The model under review builds one solid part; all positions refer to its coordinate system, in mm. A direction names the side the tool comes from. Give positions to 0.01 mm unless a question says otherwise; leave off trailing zeros. Order: outer loops, then holes, each group sorted by start corner. A loop starts at its lowest first (then second) coordinate and runs counter-clockwise, first axis right, second up. Notation, with made-up numbers: (58.5, -7.5) - (83.5, -7.5) arc R23 ccw to (83.5, 18.5) - close; hole circle Ø8 at (14.25, 61). An arc over 180 degrees is marked (long way). Answer as CSV lines item,"result". Start each with the question number.
from build123d import *

# Parameters (mm, degrees)
F0_W     = 152.4
F0_H     = 76.2
F1_DEPTH = 12.7
F2_R     = 6.35
F2_R_2   = 5.9938939969
F2_R_3   = 6.6713502792
F2_R_4   = 7.8689754044
F3_DEPTH = 12.7
F4_W     = 25.4
F4_H     = 50.8
F6_W     = 17.78
F6_H     = 17.78
F8_R     = 5.08
F9_SIZE  = 5.08


with BuildPart() as f1:
    # F0 (on Top) → F1 (new body)
    with BuildSketch(Plane.XY):
        Rectangle(F0_W, F0_H)
    extrude(amount=F1_DEPTH)

    # F2 (on Top) → F3 (cut)
    with BuildSketch(Plane.XY):
        with Locations((-67.2256079361, 27.7522747686)):
            Circle(F2_R)
        with Locations((-68.6647296343, -27.1399345782)):
            Circle(F2_R_2)
        with Locations((60.0338615502, 30.0137525229)):
            Circle(F2_R_3)
        with Locations((64.9679941536, -26.7287574834)):
            Circle(F2_R_4)
    extrude(amount=F3_DEPTH, mode=Mode.SUBTRACT)

    # F4 (on Front) → F5 (revolve)
    with BuildSketch(Plane.XZ):
        with Locations((-12.7, 38.1)):
            Rectangle(F4_W, F4_H)
    revolve(axis=Axis((0, 0, 38.1), (0, 0, -1)))

    # F6 (on Front) → F7 (revolve, cut)
    with BuildSketch(Plane.XZ):
        with Locations((21.59, 41.91)):
            Rectangle(F6_W, F6_H)
    revolve(axis=Axis((0, 0, 63.5), (0, 0, -1)), mode=Mode.SUBTRACT)

    # F8
    f8_edges = [f1.edges().sort_by_distance(p)[0] for p in [
        (25.4, 0, 63.5),
        (25.4, 0, 12.7),
    ]]
    fillet(f8_edges, radius=F8_R)

    # F9
    f9_edges = [f1.edges().sort_by_distance(p)[0] for p in [
        (25.4, 0, 33.02),
        (25.4, 0, 50.8),
    ]]
    chamfer(f9_edges, length=F9_SIZE)


solid = f1.part
Item 1: For line 1 along Z through (x, y) = (45.5, -10); line 2 along X through (y, z) = (26.5, 4); line 3 along Z through (x, y) = (-15.5, 9.5), list the stretches that pass through material, from the lowest coordinate up.
Item 2: Machinability: for faces 5 (the face through (5.506, -24.796, 57.168)), 6 (the face through (-1, -38.1, 6)), 7 (the face through (0, 13, 33.02)), which of the approach directions +Z, -Z, +X, -X, +Y, -Y give a long, thin tool a straight path to every point of the face, cutting with its end or side? Answer none if there is none.
Item 3: Clearance check with flat-ended pins moving along their axes: pin 1 (10 mm diameter, centred on x = -53.5, y = 12, fed in from +Z); pin 2 (20.5 mm diameter, centred on x = -0.5, y = 2, fed in from -Z); pin 3 (10 mm diameter, centred on y = 14.5, z = 49, fed in from +X); pin 4 (1.5 mm diameter, centred on x = -4.5, z = 27, fed in from +Y). State where each tip first meets the part, or that it passes through.
Item 4: Take a section at A-A on y = 32. Write out the cut boundary in (x, z), and give its area (3 significant figures).
Item 5: Take a section at B-B on x = 55.5. Write out the cut boundary in (y, z).
Item 6: Mouldability with a two-part tool opening along X and no side actions: class faces 1 (the face through (-1, 38.1, 6)), 2 (the face through (-65.442, -22.086, 6.261)), 3 (the face through (5.506, -24.796, 22.931)), 4 (the face through (76.2, -1, 6)) as released by +X, released by -X, zero draft, split by the parting line, or undercut.
Item 7: Take a section at D-D on y = 0. Write out the cut boundary in (x, z), and give its area (3 significant figures).
Item 8: Take a section at C-C on x = 0. Write out the cut boundary in (y, z), and give its area (3 significant figures).
Data:
1,line 1,"z = 0 to 12.7"
1,line 2,"x = -76.2 to -73.45, -61 to 54.36, 65.7 to 76.2"
1,line 3,"z = 0 to 33.02, 50.8 to 63.5"
2,face 5,"+Z"
2,face 6,"+Z, -Z, +X, -X, -Y"
2,face 7,"none"
3,pin 1,"stops at z = 12.7"
3,pin 2,"stops at z = 0"
3,pin 3,"stops at x = 19.45"
3,pin 4,"stops at y = 25.12"
4,outline,"(-76.2, 0) - (-71.95, 0) - (-71.95, 12.7) - (-76.2, 12.7) - close; (-62.51, 0) - (53.67, 0) - (53.67, 12.7) - (-62.51, 12.7) - close; (66.4, 0) - (76.2, 0) - (76.2, 12.7) - (66.4, 12.7) - close"
4,area,"1,650 mm^2"
5,outline,"(-38.1, 0) - (25.12, 0) - (25.12, 12.7) - (-38.1, 12.7) - close; (34.91, 0) - (38.1, 0) - (38.1, 12.7) - (34.91, 12.7) - close"
6,face 1,"zero draft"
6,face 2,"undercut"
6,face 3,"split by the parting line"
6,face 4,"released by +X"
7,outline,"(-76.2, 0) - (76.2, 0) - (76.2, 12.7) - (30.48, 12.7) arc R5.08 cw to (25.4, 17.78) - (25.4, 27.94) - (20.32, 33.02) - (12.7, 33.02) - (12.7, 50.8) - (20.32, 50.8) - (25.4, 55.88) - (25.4, 58.42) arc R5.08 ccw to (20.32, 63.5) - (-20.32, 63.5) arc R5.08 ccw to (-25.4, 58.42) - (-25.4, 55.88) - (-20.32, 50.8) - (-12.7, 50.8) - (-12.7, 33.02) - (-20.32, 33.02) - (-25.4, 27.94) - (-25.4, 17.78) arc R5.08 cw to (-30.48, 12.7) - (-76.2, 12.7) - close"
7,area,"4,010 mm^2"
8,outline,"(-38.1, 0) - (38.1, 0) - (38.1, 12.7) - (30.48, 12.7) arc R5.08 cw to (25.4, 17.78) - (25.4, 27.94) - (20.32, 33.02) - (12.7, 33.02) - (12.7, 50.8) - (20.32, 50.8) - (25.4, 55.88) - (25.4, 58.42) arc R5.08 ccw to (20.32, 63.5) - (-20.32, 63.5) arc R5.08 ccw to (-25.4, 58.42) - (-25.4, 55.88) - (-20.32, 50.8) - (-12.7, 50.8) - (-12.7, 33.02) - (-20.32, 33.02) - (-25.4, 27.94) - (-25.4, 17.78) arc R5.08 cw to (-30.48, 12.7) - (-38.1, 12.7) - close"
8,area,"3,050 mm^2"
